```python
from build123d import *

# Parameters (mm, degrees)
SKETCH1_R                  = 28
SKETCH1_R_2                = 26
BOSS_EXTRUDE1_DEPTH        = 8
SKETCH3_R                  = 24
BOSS_EXTRUDE2_DEPTH        = 3
SKETCH5_R                  = 2
BOSS_EXTRUDE3_DEPTH        = 11.75
BOSS_EXTRUDE3_DEPTH_BACK   = 2.5
BOSS_EXTRUDE3_2_DEPTH      = 11.75
BOSS_EXTRUDE3_2_DEPTH_BACK = 2.5
SKETCH10_R                 = 28
BOSS_EXTRUDE4_DEPTH        = 3
SKETCH16_R                 = 3
BOSS_EXTRUDE5_DEPTH        = 9.75
SKETCH20_R                 = 1.5
CUT_EXTRUDE2_DEPTH         = 30
SKETCH21_R                 = 2.5
CUT_EXTRUDE3_DEPTH         = 1


with BuildPart() as part:
    # Sketch1 → Boss-Extrude1 (new body)
    with BuildSketch(Plane(origin=(0, 0, 0), x_dir=(1, 0, 0), z_dir=(0, 1, 0))):
        Circle(SKETCH1_R)
        Circle(SKETCH1_R_2, mode=Mode.SUBTRACT)
    extrude(amount=BOSS_EXTRUDE1_DEPTH)



with BuildPart() as body_2:
    # Sketch3 → Boss-Extrude2 (new body)
    with BuildSketch(Plane(origin=(0, 0, 0), x_dir=(1, 0, 0), z_dir=(0, 1, 0))):
        Circle(SKETCH3_R)
    extrude(amount=BOSS_EXTRUDE2_DEPTH)


with BuildPart() as body_3:
    # Sketch5 → Boss-Extrude3 (new body, two sides)
    with BuildSketch(Plane(origin=(0, 3, 0), x_dir=(1, 0, 0), z_dir=(0, 1, 0))) as boss_extrude3_sk:
        with Locations((-20.2, 0)):
            Circle(SKETCH5_R)
    extrude(amount=BOSS_EXTRUDE3_DEPTH)
    extrude(boss_extrude3_sk.sketch, amount=-BOSS_EXTRUDE3_DEPTH_BACK)


with BuildPart() as body_4:
    # Sketch5 → Boss-Extrude3 2 (new body, two sides)
    with BuildSketch(Plane(origin=(0, 3, 0), x_dir=(1, 0, 0), z_dir=(0, 1, 0))) as boss_extrude3_2_sk:
        with Locations((20.2, 0)):
            Circle(SKETCH5_R)
    extrude(amount=BOSS_EXTRUDE3_2_DEPTH)
    extrude(boss_extrude3_2_sk.sketch, amount=-BOSS_EXTRUDE3_2_DEPTH_BACK)


with BuildPart() as part_1:
    add(part.part)

    add(body_2.part)  # Boss-Extrude4 merges body 2

    add(body_3.part)  # Boss-Extrude4 merges body 3

    add(body_4.part)  # Boss-Extrude4 merges body 4
    # Sketch10 → Boss-Extrude4 (add)
    with BuildSketch(Plane(origin=(0, 0, 0), x_dir=(-1, 0, 0), z_dir=(0, -1, 0))):
        Circle(SKETCH10_R)
    extrude(amount=-BOSS_EXTRUDE4_DEPTH)

    # Sketch16 → Boss-Extrude5 (add)
    with BuildSketch(Plane(origin=(0, 3, 0), x_dir=(1, 0, 0), z_dir=(0, 1, 0))):
        with Locations((20.2, 0)):
            Circle(SKETCH16_R)
        with Locations((-20.2, 0)):
            Circle(SKETCH16_R)
    extrude(amount=BOSS_EXTRUDE5_DEPTH)

    # Sketch20 → Cut-Extrude2 (cut)
    with BuildSketch(Plane(origin=(0, 14.75, 0), x_dir=(1, 0, 0), z_dir=(0, 1, 0))):
        with Locations((20.2, 0)):
            Circle(SKETCH20_R)
        with Locations((-20.2, 0)):
            Circle(SKETCH20_R)
    extrude(amount=-CUT_EXTRUDE2_DEPTH, mode=Mode.SUBTRACT)

    # Sketch21 → Cut-Extrude3 (cut)
    with BuildSketch(Plane.XZ):
        with Locations((20.2, 0)):
            Circle(SKETCH21_R)
        with Locations((-20.2, 0)):
            Circle(SKETCH21_R)
    extrude(amount=-CUT_EXTRUDE3_DEPTH, mode=Mode.SUBTRACT)


solid = part_1.part
```
CAD build for the part. Positions are in the model's coordinates, mm. A direction names the side the tool comes from. Coordinates: 2 decimals unless noted, no trailing zeros. Order: outer loops, then holes, each group sorted by start corner. A loop starts at its lowest first (then second) coordinate and runs counter-clockwise, first axis right, second up.
(1) Mould opens along Z. For faces 4 (the face through (-22, 14.75, 0)), 5 (the face through (25.865, 3.944, 10.724)), 6 (the face through (-20.633, 5.465, 15.821)) say: released by +Z, released by -Z, zero draft, split by the parting line, or undercut.
Solution:
face 4: zero draft
face 5: split by the parting line
face 6: undercut
(2) Which spindle directions (+Z, -Z, +X, -X, +Y, -Y) get a long thin tool onto all of the face, cutting with end or side? Do faces 1 (the face through (22.97, 7.81, 1.15)), 2 (the face through (0, 0, 0)), 3 (the face through (-20, 1, -2)). Say none if no direction does.
Solution:
face 1: +Y
face 2: +Z, -Z, +X, -X, -Y
face 3: -Y
(3) Saw through at D-D, the plane z = -12.5. Write the cut outline in (x, y).
Solution:
outline: (-25.05, 0) - (25.05, 0) - (25.05, 8) - (22.8, 8) - (22.8, 3) - (-22.8, 3) - (-22.8, 8) - (-25.05, 8) - close
(4) Saw through at A-A, the plane y = 7. Write the cut outline in (x, z).
Solution:
outline: circle Ø56 at (0, 0); circle Ø6 at (-20.2, 0); circle Ø6 at (20.2, 0); hole circle Ø52 at (0, 0); hole circle Ø3 at (-20.2, 0); hole circle Ø3 at (20.2, 0)
(5) Drill centre lines: L1, parallel to Z at x = -20.2, y = 8.5; L2, parallel to X at y = 4.25, z = 0; L3, parallel to Z at x = -18.5, y = 6.25. Where is each one in solid material? Low to high.
Solution:
L1: z = -3 to -1.5, 1.5 to 3
L2: x = -28 to -26, -23.2 to -21.7, -18.7 to -17.2, 17.2 to 18.7, 21.7 to 23.2, 26 to 28
L3: z = -21.02 to -18.27, -2.47 to 2.47, 18.27 to 21.02
(6) Saw through at B-B, the plane y = 13.5. Write the cut outline in (x, z).
Solution:
outline: circle Ø4 at (-20.2, 0); circle Ø4 at (20.2, 0); hole circle Ø3 at (-20.2, 0); hole circle Ø3 at (20.2, 0)
(7) Saw through at C-C, the plane x = -20.2. Write the cut outline in (y, z), and give its area (3 significant figures).
Solution:
outline: (0, -19.39) - (8, -19.39) - (8, -16.37) - (3, -16.37) - (3, -3) - (12.75, -3) - (12.75, -2) - (14.75, -2) - (14.75, -1.5) - (1, -1.5) - (1, -2.5) - (0, -2.5) - close; (0, 2.5) - (1, 2.5) - (1, 1.5) - (14.75, 1.5) - (14.75, 2) - (12.75, 2) - (12.75, 3) - (3, 3) - (3, 16.37) - (8, 16.37) - (8, 19.39) - (0, 19.39) - close
area: 167 mm2
(8) Pin check, flat tips, straight feed: pin 1 Ø3.5 at (x, z) = (20.2, 0) entering from -Y; pin 2 Ø6 at (y, z) = (10.5, -4.5) entering from -X; pin 3 Ø4 at (x, z) = (-0.5, -17.5) entering from +Y. Stop position of each tip, or through.
Solution:
pin 1: stops at y = 1
pin 2: stops at x = -27.86
pin 3: stops at y = 3
